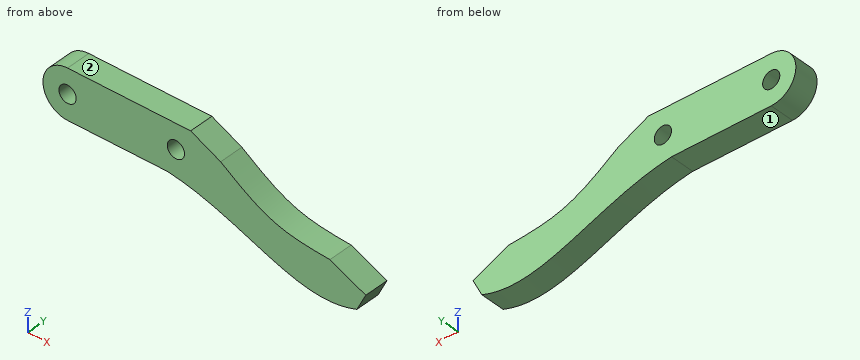
```python
from build123d import *

# Parameters (mm, degrees)
SKETCH1_R           = 5
SKETCH1_R_2         = 1.75
BOSS_EXTRUDE1_DEPTH = 5
BOSS_EXTRUDE2_START = -5
BOSS_EXTRUDE2_DEPTH = 5


with BuildPart() as part:
    # Sketch1 → Boss-Extrude1 (new body)
    # profile 1 of 3: a face of its own
    with BuildSketch(Plane(origin=(0, 0, 0), x_dir=(1, 0, 0), z_dir=(0, 1, 0))):
        Circle(SKETCH1_R)
        with Locations(Location((0, 0, 0), (0, 0, 270))):
            Circle(SKETCH1_R_2, mode=Mode.SUBTRACT)
    # profile 2 of 3: a face of its own
    with BuildSketch(Plane(origin=(0, 0, 0), x_dir=(1, 0, 0), z_dir=(0, 1, 0))):
        with BuildLine():
            Line((22, 5), (7e-09, 5))
            ThreePointArc((7e-09, 5), (3.535533908, 3.535533903), (5, 0))
            ThreePointArc((5, 0), (3.535533907, -3.535533905), (3e-09, -5))
            Line((3e-09, -5), (22, -5))
            ThreePointArc((22, -5), (17, 0), (22, 5))
        make_face()
    # profile 3 of 3: a face of its own
    with BuildSketch(Plane(origin=(0, 0, 0), x_dir=(1, 0, 0), z_dir=(0, 1, 0))):
        with Locations((22, 0)):
            Circle(SKETCH1_R)
        with Locations(Location((22, 0, 0), (0, 0, 270))):
            Circle(SKETCH1_R_2, mode=Mode.SUBTRACT)
    extrude(amount=BOSS_EXTRUDE1_DEPTH)

    # Sketch2 → Boss-Extrude2 (add)
    with BuildSketch(Plane(origin=(0, 5, 0), x_dir=(1, 0, 0), z_dir=(0, 1, 0)).offset(BOSS_EXTRUDE2_START)):
        with BuildLine():
            ThreePointArc((22, 5), (27, 0), (22, -5))
            Line((22, -5), (24.99, -5))
            Line((24.99, -5), (31.08, -2.029708536))
            add(Edge.make_bspline(
                [(31.08, -2.029708536), (34.749760943, 0.550345092), (41.451086478, 5.261763501), (49.588688562, 5.770056828), (53.27, 6)],
                knots=[0, 0, 0, 0, 0.547617173, 1, 1, 1, 1], degree=3))
            Line((53.27, 6), (60.557013712, 9.301428655))
            Line((60.557013712, 9.301428655), (58.75, 12.87))
            add(Edge.make_bspline(
                [(20.251877892, 5), (35.741313443, 6.892403077), (46.679161054, 17.378023899), (58.75, 12.87)],
                knots=[0.158187399, 0.158187399, 0.158187399, 0.158187399, 1, 1, 1, 1], degree=3))
            Line((20.251877892, 5), (22, 5))
        make_face()
    extrude(amount=BOSS_EXTRUDE2_DEPTH)


solid = part.part
```
Geometry check sheet. Reference: the model listing, model coordinates, mm. Face numbers are marked on the shaded views. A direction names the side the tool comes from. Coordinates: 2 decimals unless noted, no trailing zeros. Order: outer loops, then holes, each group sorted by start corner. A loop starts at its lowest first (then second) coordinate and runs counter-clockwise, first axis right, second up. Notation, with made-up numbers: (10.25, 0.5) - (45.25, 0.5) arc R17 ccw to (45.25, 20.5) - close; hole circle Ø9 at (15.25, -10.5). An arc over 180 degrees is marked (long way). Use one line per item in the form item = value.
1. Scan lines: line 1 (X direction, y = 2.95, z = 0); line 2 (X direction, y = 0.65, z = 1); line 3 (Z direction, x = 5.5, y = 2.6). Record each from-to range of solid material in increasing order.
Here are the results:
line_1 = -5 to -1.75, 1.75 to 20.25, 23.75 to 34.01
line_2 = -4.9 to -1.44, 1.44 to 20.56, 23.44 to 32.55
line_3 = -5 to 5
2. Section check B-B (z = 0). State how many separate pieces and enclosed holes the cut face has, then the cut area to 3 significant figures.
Here are the results:
separate_pieces = 3
enclosed_holes = 0
area = 160 mm²
3. Access from +Z, -Z, +X, -X, +Y, -Y to the whole of each face (thin tool, end or side, straight path). Record for the marked faces 1 and 2.
Here are the results:
face_1 = -Z, -X, +Y, -Y
face_2 = +Z, +X, -X, +Y, -Y
4. Section check A-A (x = 16.5). Record the boundary of the cut face in (y, z), then the cut area to 3 significant figures.
Here are the results:
outline = (0, -5) - (5, -5) - (5, 5) - (0, 5) - close
area = 50.0 mm²
5. Gauge pin test, flat ends, axial feed: pin 1 (1.5 mm diameter, centred on y = 1, z = 2.5, fed in from +X); pin 2 (3 mm diameter, centred on x = 28.5, y = 1.5, fed in from -Z); pin 3 (2.5 mm diameter, centred on x = 7.5, y = 3, fed in from -Z). Record the tip position at first contact, or that the pin passes through.
Here are the results:
pin_1 = 31.48
pin_2 = -7.29
pin_3 = -5
